Can you work these out from the drawing? Everything is in mm from the part's minimum corner. Round coordinates to 2 decimals unless told otherwise and drop trailing zeros. Order: outer loops, then holes, each group sorted by start corner. A loop starts at its lowest first (then second) coordinate and runs counter-clockwise, first axis right, second up. Notation, with made-up numbers: (42, -27) -> (92, -27) arc R29 cw to (92, 12) -> close; hole circle Ø10 at (54, -21.5). An arc over 180 degrees is marked (long way). One line per item, written item: value.
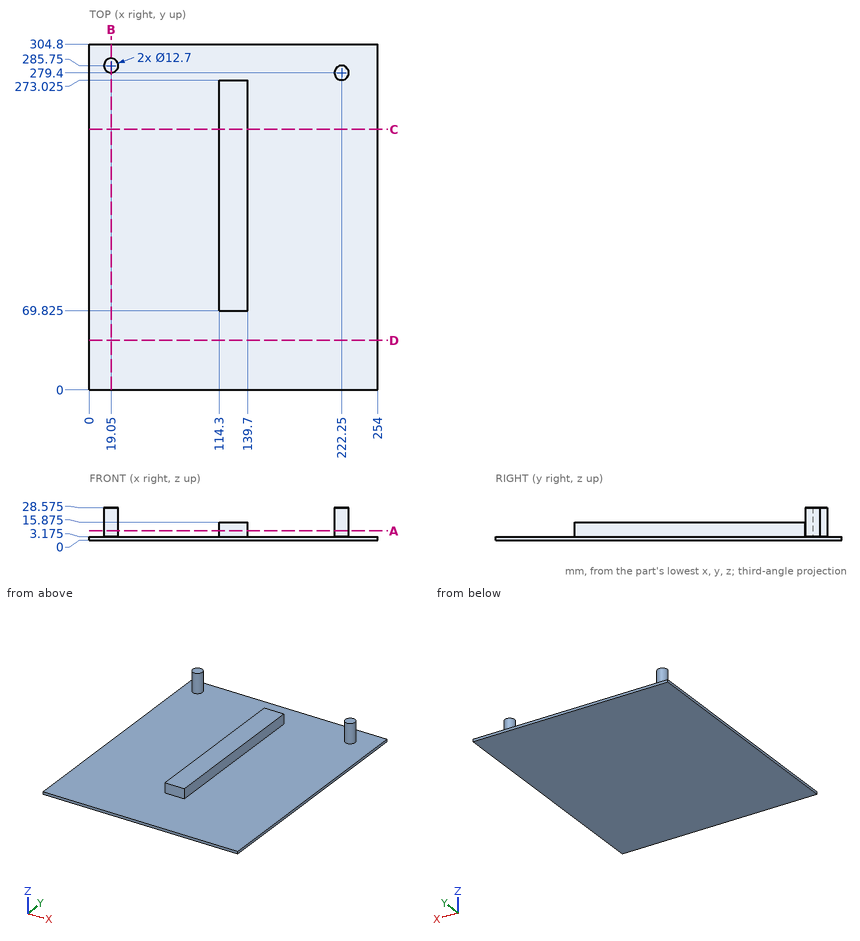
Q1. I want a section at D-D on y = 43.5. List the corners of the cut face in (x, z) for me (1 decimal).
Answers below:
outline: (0, 0) -> (254, 0) -> (254, 3.2) -> (0, 3.2) -> close
Q2. I want a section at A-A on z = 8.25. Give the number of separate pieces and of enclosed holes in the cut face.
Answers below:
separate pieces: 3
enclosed holes: 0
Q3. Will these pins go through, and if not, where does the flat tip stop? pin 1 Ø8 at (x, z) = (196, 9) entering from +Y; pin 2 Ø7.5 at (x, y) = (127.5, 149.5) entering from +Z (3 decimals); pin 3 Ø1 at (x, y) = (226, 251) entering from +Z (3 decimals); pin 4 Ø5 at (y, z) = (135.5, 17) entering from -X.
Answers below:
pin 1: through
pin 2: z = 15.875
pin 3: z = 3.175
pin 4: x = 114.3
Q4. Please list where these lines run through material, in increasing order: line 1 along Z through (x, y) = (164, 61.5) (1 decimal); line 2 along X through (y, z) = (239.5, 9); line 3 along Y through (x, z) = (219.5, 11.25) (1 decimal).
Answers below:
line 1: 0 to 3.2
line 2: 114.3 to 139.7
line 3: 273.7 to 285.1
Q5. I want a section at B-B on x = 19.05. List the corners of the cut face in (y, z) for me (1 decimal), plus the area to 3 significant figures.
Answers below:
outline: (0, 0) -> (304.8, 0) -> (304.8, 3.2) -> (292.1, 3.2) -> (292.1, 28.6) -> (279.4, 28.6) -> (279.4, 3.2) -> (0, 3.2) -> close
area: 1,290 mm^2
Q6. I want a section at C-C on y = 229.5. List the corners of the cut face in (x, z) for me (1 decimal), plus the area to 3 significant figures.
Answers below:
outline: (0, 0) -> (254, 0) -> (254, 3.2) -> (139.7, 3.2) -> (139.7, 15.9) -> (114.3, 15.9) -> (114.3, 3.2) -> (0, 3.2) -> close
area: 1,130 mm^2
